from build123d import *

# Parameters (mm, degrees)
F1_DEPTH = 10
F0_W     = 36.4919372275
F0_H     = 8
F2_DEPTH = 3
F3_ANGLE = 22.5
F4_R     = 1.5
F5_DEPTH = 28.001


with BuildPart() as f1:
    # F0 (on Top) → F1 (new body)
    with BuildSketch(Plane.XY):
        Polygon((26.5120977908, 10), (-17.4879022092, 10), (-17.4879022092, -18), (26.5120977908, -18), (26.5120977908, -10), (-9.9798394367, -10), (-9.9798394367, -8), (-9.9798394367, 0), (-9.9798394367, 2), (26.5120977908, 2), align=None)
    extrude(amount=-F1_DEPTH)

    # F0 (on Top) → F2 (join)
    with BuildSketch(Plane.XY):
        with Locations((8.2661291771, -4)):
            Rectangle(F0_W, F0_H)
    extrude(amount=-F2_DEPTH)

    # F0 (on Top) → F3 (revolve)
    with BuildSketch(Plane.XY):
        with Locations((8.2661291771, -4)):
            Rectangle(F0_W, F0_H)
    revolve(axis=Axis((-9.9798394367, -4, 0), (0, -1, 0)), revolution_arc=F3_ANGLE)

    # F4 (on face) → F5 (cut, through all)
    with BuildSketch(Plane.XZ.offset(18)):
        with Locations((-11.4879022092, -5)):
            Circle(F4_R)
        with Locations((4.5120977908, -5)):
            Circle(F4_R)
        with Locations((20.5120977908, -5)):
            Circle(F4_R)
    extrude(amount=-F5_DEPTH, mode=Mode.SUBTRACT)


solid = f1.part
The listing builds one solid part. Answer for the finished solid, in the listing's coordinates (mm). A direction names the side the tool comes from. Give positions to 0.01 mm unless a question says otherwise; leave off trailing zeros. Order: outer loops, then holes, each group sorted by start corner. A loop starts at its lowest first (then second) coordinate and runs counter-clockwise, first axis right, second up. Notation, with made-up numbers: (36, 63.5) - (68, 63.5) arc R19 ccw to (68, 82.5) - close; hole circle Ø10 at (57.5, 29.5). An arc over 180 degrees is marked (long way). One line per item, written item: value. Start each with the question number.
1) A cutting plane is placed at D-D on x = -4.5. Give the vertices of the cut face in (y, z).
2) The mould has two halves that part along Z. Classify faces 3 (the face through (8, -4, -3)), 4 (the face through (25.83, -3.94, 7.02)), 5 (the face through (19.014, -14.056, -4.934)): released by +Z, released by -Z, zero draft, split by the parting line, or undercut.
3) Find the intervals of material crossed by L1, parallel to Y at x = 13, z = -1; L2, parallel to Y at x = -7.5, z = -8.25; L3, parallel to X at y = 5.25, z = -4.75, in increasing order.
4) A cutting plane is placed at C-C on x = 10.5. Give the vertices of the cut face in (y, z), then the cut area to 3 significant figures.
5) A cutting plane is placed at A-A on z = -5. Give the vertices of the cut face in (x, y), then the cut area to 3 significant figures.
6) Given pin 1 Ø2 at (x, y) = (3, 3.5) entering from +Z; pin 2 Ø5 at (x, z) = (6, 2) entering from -Y; pin 3 Ø9 at (x, y) = (0, -3) entering from -Z; pin 4 Ø1 at (x, y) = (7, -3.5) entering from +Z, each flat-ended and moving along its own axis, determine where each tip first touches the part or whether it passes through.
7) A cutting plane is placed at B-B on y = -12.5. Give the vertices of the cut face in (x, z).
8) A tool of negligible diameter and unlimited length cuts with its end or side. For faces 1 (the face through (5.943, 5.944, -4.549)), 2 (the face through (8, 2, -5)), from which of +Z, -Z, +X, -X, +Y, -Y can it reach the whole face along a straight path? Write none if from no direction.
Answer sheet:
1. outline: (-18, -10) - (-10, -10) - (-10, 0) - (-18, 0) - close; (-8, -3) - (0, -3) - (0, 2.27) - (-8, 2.27) - close; (2, -10) - (10, -10) - (10, 0) - (2, 0) - close
2. face 3: released by -Z
2. face 4: released by +Z
2. face 5: undercut
3. L1: y = -18 to -10, -8 to 0, 2 to 10
3. L2: y = -18 to -10, 2 to 10
3. L3: x = -17.49 to -12.97, -10.01 to 3.03, 5.99 to 19.03, 21.99 to 26.51
4. outline: (-18, -10) - (-10, -10) - (-10, 0) - (-18, 0) - close; (-8, -3) - (0, -3) - (0, 8.48) - (-8, 8.48) - close; (2, -10) - (10, -10) - (10, 0) - (2, 0) - close
4. area: 252 mm2
5. outline: (-17.49, -18) - (-12.99, -18) - (-12.99, 10) - (-17.49, 10) - close; (-9.99, -18) - (3.01, -18) - (3.01, -10) - (-9.98, -10) - (-9.98, 2) - (3.01, 2) - (3.01, 10) - (-9.99, 10) - close; (6.01, -18) - (19.01, -18) - (19.01, -10) - (6.01, -10) - close; (6.01, 2) - (19.01, 2) - (19.01, 10) - (6.01, 10) - close; (22.01, -18) - (26.51, -18) - (26.51, -10) - (22.01, -10) - close; (22.01, 2) - (26.51, 2) - (26.51, 10) - (22.01, 10) - close
5. area: 614 mm2
6. pin 1: stops at z = 0
6. pin 2: stops at y = -18
6. pin 3: stops at z = -3
6. pin 4: stops at z = 7.24
7. outline: (-17.49, -10) - (26.51, -10) - (26.51, 0) - (-17.49, 0) - close; hole circle Ø3 at (-11.49, -5); hole circle Ø3 at (4.51, -5); hole circle Ø3 at (20.51, -5)
8. face 1: +Y, -Y
8. face 2: +Z, -Z, +X
